from build123d import *

# Parameters (mm, degrees)
BOSS_EXTRUDE1_DEPTH = 14.5
CUT_EXTRUDE1_DEPTH  = 3.6
CUT_EXTRUDE2_DEPTH  = 3.6
CUT_EXTRUDE3_START  = -2
SKETCH4_R           = 3.0000000000000004
SKETCH4_R_2         = 1.75
CUT_EXTRUDE3_DEPTH  = 1.6
SKETCH5_R           = 2
CUT_EXTRUDE4_DEPTH  = 5
FILLET1_R           = 0.5
FILLET3_R           = 0.5
SKETCH6_W           = 0.7512194361763478
SKETCH6_H           = 6
CUT_EXTRUDE5_DEPTH  = 1
SKETCH7_W           = 7.9403086641005265
SKETCH7_H           = 0.6946760377543701
CUT_EXTRUDE6_DEPTH  = 1
SKETCH8_R           = 1.75
BOSS_EXTRUDE2_DEPTH = 7


with BuildPart() as part:
    # Sketch1 → Boss-Extrude1 (new body)
    with BuildSketch(Plane(origin=(0, 0, 0), x_dir=(1, 0, 0), z_dir=(0, 1, 0))):
        Polygon((-3.0000000000000004, 3), (2.9999999999999996, 3), (3.0000000000000004, -3), (-2.9999999999999996, -3), align=None)
    extrude(amount=BOSS_EXTRUDE1_DEPTH)

    # Sketch2 → Cut-Extrude1 (cut)
    with BuildSketch(Plane(origin=(0, 14.5, 0), x_dir=(1, 0, 0), z_dir=(0, 1, 0))):
        Polygon((2, 3), (-2, 3), (-2, -3), (2, -2.9999999999999982), align=None)
    extrude(amount=-CUT_EXTRUDE1_DEPTH, mode=Mode.SUBTRACT)

    # Sketch3 → Cut-Extrude2 (cut)
    with BuildSketch(Plane.XZ):
        with BuildLine():
            ThreePointArc((-4.6684e-13, -3), (-2.121320343559808, -2.1213203435594776), (-3, 3.7e-16))
            Line((-2.9999999999999996, -2.22e-15), (-2.9999999999999996, -3))
            Line((-2.9999999999999996, -3), (-4.6674e-13, -3))
        make_face()
        with BuildLine():
            Line((2.9999999999999996, -3), (2.9999999999999996, 0))
            ThreePointArc((3, -7.3e-16), (2.121320343559478, -2.121320343559807), (-4.6684e-13, -3))
            Line((-4.6674e-13, -3), (2.9999999999999996, -3))
        make_face()
        with BuildLine():
            Line((2.9999999999999996, 3), (-4.6763e-13, 3))
            ThreePointArc((-4.6678e-13, 3), (2.1213203435594776, 2.1213203435598076), (3, 0))
            Line((2.9999999999999996, 0), (2.9999999999999996, 3))
        make_face()
        with BuildLine():
            Line((-4.6763e-13, 3), (-2.9999999999999996, 3))
            Line((-2.9999999999999996, 3), (-2.9999999999999996, -2.22e-15))
            ThreePointArc((-3, 3.7e-16), (-2.121320343559808, 2.1213203435594767), (-4.6744e-13, 3))
        make_face()
    extrude(amount=-CUT_EXTRUDE2_DEPTH, mode=Mode.SUBTRACT)

    # Sketch4 → Cut-Extrude3 (cut)
    with BuildSketch(Plane.XZ.offset(CUT_EXTRUDE3_START)):
        with Locations(Location((0, 0, 0), (0, 0, 270))):
            Circle(SKETCH4_R)
        with Locations(Location((0, 0, 0), (0, 0, 270))):
            Circle(SKETCH4_R_2, mode=Mode.SUBTRACT)
    extrude(amount=-CUT_EXTRUDE3_DEPTH, mode=Mode.SUBTRACT)

    # Sketch5 → Cut-Extrude4 (cut)
    with BuildSketch(Plane.XY.offset(3)):
        with Locations((0, 7.249999999999999)):
            Circle(SKETCH5_R)
    extrude(amount=-CUT_EXTRUDE4_DEPTH, mode=Mode.SUBTRACT)

    # Fillet1
    fillet1_edges = [part.edges().sort_by_distance(p)[0] for p in [
        (-3, 0, 5.9e-16),
        (-3.0000000000000004, 2, 3.82e-15),
    ]]
    fillet(fillet1_edges, radius=FILLET1_R)

    # Fillet3
    fillet3_edges = [part.edges().sort_by_distance(p)[0] for p in [
        (-3, 14.5, 0),
        (-2.5, 14.5, -3),
        (2.5, 14.5, 3),
        (-2.4999999999999996, 14.5, 3),
        (-2, 12.7, 3),
        (0, 10.9, -3),
        (-2, 12.7, -3),
        (2, 12.7, -3),
        (0, 10.9, 2.999999999999999),
        (2, 12.7, 2.9999999999999982),
        (0, 3.6, 3),
        (2.9999999999999996, 3.6, 0),
        (3, 14.5, 0),
        (0, 3.6, -3),
        (-2.9999999999999996, 3.6, 0),
        (3.0000000000000004, 9.05, 3),
        (-2.9999999999999996, 9.05, 3),
        (-3.0000000000000004, 9.05, -3),
        (2.9999999999999996, 9.05, -3),
        (2.4999999999999996, 14.5, -3),
        (-2, 7.249999999999999, 3),
    ]]
    fillet(fillet3_edges, radius=FILLET3_R - 0.0001)  # a hair under: the kernel refuses the full size

    # Sketch6 → Cut-Extrude5 (cut)
    with BuildSketch(Plane.XZ):
        Rectangle(SKETCH6_W, SKETCH6_H)
    extrude(amount=-CUT_EXTRUDE5_DEPTH, mode=Mode.SUBTRACT)

    # Sketch7 → Cut-Extrude6 (cut)
    with BuildSketch(Plane.XZ):
        Rectangle(SKETCH7_W, SKETCH7_H)
    extrude(amount=-CUT_EXTRUDE6_DEPTH, mode=Mode.SUBTRACT)

    # Sketch8 → Boss-Extrude2 (add)
    with BuildSketch(Plane.XZ.offset(-1)):
        with Locations(Location((0, 0, 0), (0, 0, 270))):
            Circle(SKETCH8_R)
    extrude(amount=-BOSS_EXTRUDE2_DEPTH)


solid = part.part
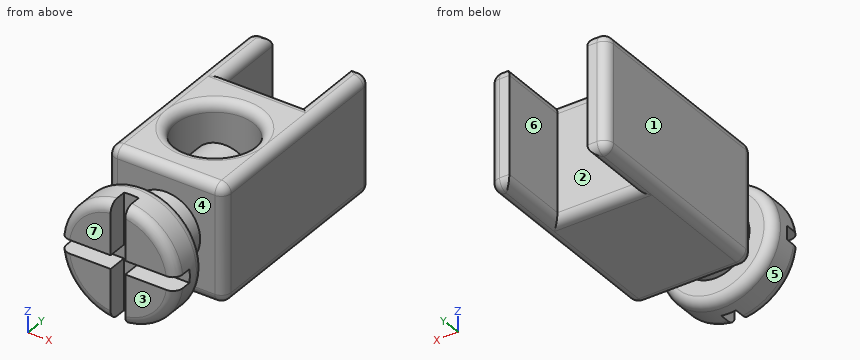
Could you check a few things on this model? Use its own coordinates, in mm. Face numbers are marked on the shaded views. A direction names the side the tool comes from. Round coordinates to 2 decimals unless told otherwise and drop trailing zeros. Order: outer loops, then holes, each group sorted by start corner. A loop starts at its lowest first (then second) coordinate and runs counter-clockwise, first axis right, second up.
Q1. Which directions (+Z, -Z, +X, -X, +Y, -Y) give clear straight access to the entire face, cutting with the end or side of a thin tool? Please do the marked faces 4, 5, 6 and 7.
Geometry says:
face 4: none
face 5: -Y
face 6: +Z, -Z, +Y
face 7: +Z, -Z, +X, -X, -Y
Q2. Imagine slicing it at B-B, the plane x = 0. List the corners of the cut face in (y, z) for me, then the cut area to 3 significant figures.
Geometry says:
outline: (1, -3) - (1.5, -3) arc R0.5 ccw to (2, -2.5) - (2, -1.75) - (3.6, -1.75) - (3.6, -2.5) arc R0.5 ccw to (4.1, -3) - (10.4, -3) arc R0.5 ccw to (10.9, -2.5) - (10.9, 2.5) arc R0.5 ccw to (10.4, 3) - (9.75, 3) arc R0.5 ccw to (9.25, 2.5) - (9.25, -2) - (5.25, -2) - (5.25, -1.75) - (8, -1.75) - (8, 1.75) - (5.25, 1.75) - (5.25, 2.5) arc R0.5 ccw to (4.75, 3) - (4.1, 3) arc R0.5 ccw to (3.6, 2.5) - (3.6, 1.75) - (2, 1.75) - (2, 2.5) arc R0.5 ccw to (1.5, 3) - (1, 3) - close
area: 44.6 mm2
Q3. Please list where these lines run through material, in increasing order: probe 1 along Y at (x, z) = (0, 1.6); probe 2 along X at (y, z) = (12.5, -2.5); probe 3 along Y at (x, z) = (0, -2.25).
Geometry says:
probe 1: y = 1 to 8, 9.25 to 10.9
probe 2: x = -3 to -2, 2 to 3
probe 3: y = 1 to 2, 3.6 to 10.9
Q4. Thinking about a two-plate mould opening in X: for the marked faces 1, 2 and 3, which applies, released by +X, released by -X, zero draft, split by the parting line, or undercut?
Geometry says:
face 1: released by -X
face 2: undercut
face 3: zero draft
Q5. Imagine slicing it at C-C, the plane z = 0. List the corners of the cut face in (x, y) for me, then the cut area to 3 significant figures.
Geometry says:
outline: (-3, 1) - (3, 1) - (3, 1.5) arc R0.5 ccw to (2.5, 2) - (1.75, 2) - (1.75, 3.6) - (2.5, 3.6) arc R0.5 ccw to (3, 4.1) - (3, 14) arc R0.5 ccw to (2.5, 14.5) - (2, 14.5) - (2, 10.9) - (-2, 10.9) - (-2, 14.5) - (-2.5, 14.5) arc R0.5 ccw to (-3, 14) - (-3, 4.1) arc R0.5 ccw to (-2.5, 3.6) - (-1.75, 3.6) - (-1.75, 2) - (-2.5, 2) arc R0.5 ccw to (-3, 1.5) - close; hole (-1.75, 6.28) - (-1.75, 8) - (1.75, 8) - (1.75, 6.28) arc R2 ccw (long way) to start
area: 58.3 mm2
Q6. I'm going to push flat-ended pins straight in: P1, Ø3, axis at x = 0.5, z = 1.5, coming from the -Y side; P2, Ø1.1, axis at x = 2, y = 0.5, coming from the +Z side; P3, Ø1.2, axis at x = 0, z = 1, coming from the +Y side; P4, Ø0.8, axis at x = 1, y = 0.5, coming from the -Z side. Where does each tip first touch, or does it pass through?
Geometry says:
P1: stops at y = 0
P2: stops at z = 2.63
P3: stops at y = 10.9
P4: stops at z = -2.94
Q7. Imagine slicing it at D-D, the plane z = 2. State how many separate pieces and enclosed holes the cut face has, then the cut area to 3 significant figures.
Geometry says:
separate pieces: 2
enclosed holes: 1
area: 46.1 mm2
